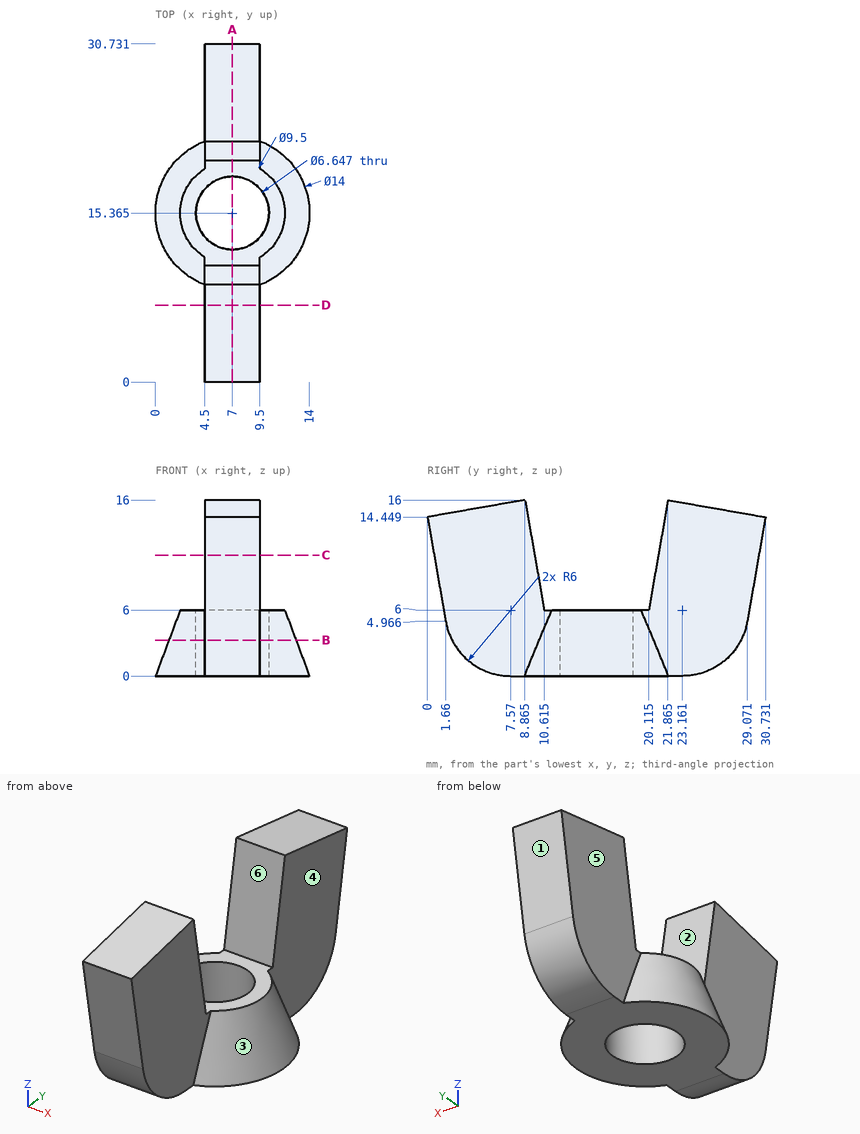
Study the drawing (mm; zero at the part's minimum x, y, z) and answer. A direction names the side the tool comes from. Give positions to 0.01 mm unless a question says otherwise; leave off trailing zeros. Order: outer loops, then holes, each group sorted by start corner. A loop starts at its lowest first (then second) coordinate and runs counter-clockwise, first axis right, second up. Notation, with made-up numbers: M -4.75,58 L 27.25,58 A15 cw 27.25,67 Z; hole C -16.5,9 d6. An arc over 180 degrees is marked long. Put each result on its own line as item: value. Start each with the question number.
Item 1: For a pull along Y with two mould halves and no side action, classify the marked faces 1, 2 and 3 as +Y half, -Y half, draft (parallel to the pull), parting line (faces both ways), or undercut.
Item 2: Flat-ended cylindrical pins translate along their axes: P1, Ø3, axis at y = 9, z = 13, coming from the +X side; P2, Ø5.5, axis at y = 26.5, z = 6.5, coming from the -X side; P3, Ø1, axis at x = 3.5, z = 12.5, coming from the +Y side; P4, Ø8, axis at y = 7.5, z = 2.5, coming from the -X side. Find the tip coordinate at first contact, or state that the pin passes through.
Item 3: Which of the six approach directions +Z, -Z, +X, -X, +Y, -Y give full straight-line access (tool end or side, diameter ignored) to the marked faces 4, 5 and 6?
Item 4: The part is cut by section C-C, the plane z = 11. Determine the outline of the cut face in (x, y).
Item 5: Find the intervals of material crossed by line 1 along X through (y, z) = (8.5, 12); line 2 along Z through (x, y) = (8.75, 12.5); line 3 along Y through (x, z) = (8.5, 10.75) (1 decimal), in increasing order.
Item 6: The part is cut by section D-D, the plane y = 7. Determine the outline of the cut face in (x, z).
Item 7: The part is cut by section B-B, the plane z = 3.25. Determine the outline of the cut face in (x, y) (1 decimal), and give its area (3 significant figures).
Item 8: The part is cut by section A-A, the plane x = 7. Determine the outline of the cut face in (y, z) (1 decimal).
Answer key:
1. face 1: +Y half
1. face 2: undercut
1. face 3: parting line
2. P1: stops at x = 9.5
2. P2: stops at x = 4.5
2. P3: passes through
2. P4: stops at x = 1.8
3. face 4: +Z, +X, +Y
3. face 5: +Z, -X, +Y
3. face 6: +Z, +X, -X
4. outline: M 4.5,0.6 L 9.5,0.6 L 9.5,9.74 L 4.5,9.74 Z; M 4.5,20.99 L 9.5,20.99 L 9.5,30.13 L 4.5,30.13 Z
5. line 1: x = 4.5 to 9.5
5. line 2: z = 0 to 6
5. line 3: y = 0.6 to 9.8, 20.9 to 30.1
6. outline: M 4.5,0.03 L 9.5,0.03 L 9.5,15.67 L 4.5,15.67 Z
7. outline: M 4.5,2.2 L 9.5,2.2 L 9.5,10.2 A5.8 ccw 9.5,20.6 L 9.5,28.5 L 4.5,28.5 L 4.5,20.6 A5.8 ccw 4.5,10.2 Z; hole C 7,15.4 d6.6
7. area: 146 mm²
8. outline: M 0,14.4 L 1.7,5 A6 ccw 7.6,0 L 12,0 L 12,6 L 10.6,6 L 8.9,16 Z; M 18.7,0 L 23.2,0 A6 ccw 29.1,5 L 30.7,14.4 L 21.9,16 L 20.1,6 L 18.7,6 Z
